Source: CAD feature listing. Evaluate the final solid. Frame: model axes, mm. A direction names the side the tool comes from. Give positions to 0.01 mm unless a question says otherwise; leave off trailing zeros. Write each loop counter-clockwise with the first axis right and the second up, starting at its lowest first coordinate (ties: lowest second). Pieces come first, ordered by that corner, then holes. Notation, with made-up numbers: (12.25, 60) -> (42.25, 60) arc R37 ccw to (42.25, 97) -> close; hole circle Ø1 at (49.25, 62). An arc over 180 degrees is marked (long way). Write item = value, one per line.
from build123d import *

# Parameters (mm, degrees)
SKETCH_2_W           = 80
SKETCH_2_H           = 34
SKETCH_2_R           = 4.05
EXTRUDE_1_DEPTH      = 8
SKETCH_3_R           = 2.55
CUT_EXTRUDE_1_DEPTH  = 88.292611371
CUT_EXTRUDE_2_DEPTH  = 88.292611371
SKETCH_5_R           = 1.55
CUT_EXTRUDE_3_DEPTH  = 88.292611371
CUT_EXTRUDE_15_DEPTH = 4.5
SKETCH_11_R          = 1.55
CUT_EXTRUDE_7_DEPTH  = 88.292611371
CUT_EXTRUDE_11_DEPTH = 2
SKETCH_21_R          = 2.9
CUT_EXTRUDE_13_DEPTH = 88.292611371
CUT_EXTRUDE_14_DEPTH = 6


with BuildPart() as part:
    # 草图2 → 凸台-拉伸1 (new body)
    with BuildSketch(Plane.XY):
        with Locations((40, 17)):
            Rectangle(SKETCH_2_W, SKETCH_2_H)
        with Locations((7, 8)):
            Circle(SKETCH_2_R, mode=Mode.SUBTRACT)
        with Locations((40, 10)):
            Circle(SKETCH_2_R, mode=Mode.SUBTRACT)
        with Locations((73, 8)):
            Circle(SKETCH_2_R, mode=Mode.SUBTRACT)
    extrude(amount=EXTRUDE_1_DEPTH)

    # 草图3 → 切除-拉伸1 (cut, through all)
    with BuildSketch(Plane.XY.offset(8)):
        with Locations((23, 8)):
            Circle(SKETCH_3_R)
        with Locations((57, 8)):
            Circle(SKETCH_3_R)
    extrude(amount=-CUT_EXTRUDE_1_DEPTH, mode=Mode.SUBTRACT)

    # 草图4 → 切除-拉伸2 (cut, through all)
    with BuildSketch(Plane(origin=(80, 0, 0), x_dir=(0, 0, -1), z_dir=(1, 0, 0))):
        Polygon((-1.5, 32.2), (-2.5, 32.2), (-2.5, 34), (0, 34), (0, 28.8), (-1.5, 28.8), align=None)
    extrude(amount=-CUT_EXTRUDE_2_DEPTH, mode=Mode.SUBTRACT)

    # 草图5 → 切除-拉伸3 (cut, through all)
    with BuildSketch(Plane.XY.offset(8)):
        with Locations((48, 10)):
            Circle(SKETCH_5_R)
        with Locations((32, 10)):
            Circle(SKETCH_5_R)
    extrude(amount=-CUT_EXTRUDE_3_DEPTH, mode=Mode.SUBTRACT)

    # 草图8 → 切除-拉伸15 (cut)
    with BuildSketch(Plane(origin=(0, 0, 0), x_dir=(-1, 0, 0), z_dir=(0, 0, -1))):
        Polygon((-48, 6.709103466), (-45.15, 8.354551733), (-45.15, 11.645448267), (-48, 13.290896534), (-50.85, 11.645448267), (-50.85, 8.354551733), align=None)
        Polygon((-34.85, 11.645448267), (-34.85, 8.354551733), (-32, 6.709103466), (-29.15, 8.354551733), (-29.15, 11.645448267), (-32, 13.290896534), align=None)
    extrude(amount=-CUT_EXTRUDE_15_DEPTH, mode=Mode.SUBTRACT)

    # 草图11 → 切除-拉伸7 (cut, through all)
    with BuildSketch(Plane(origin=(0, 0, 0), x_dir=(-1, 0, 0), z_dir=(0, 0, -1))):
        with Locations((-60, 25)):
            Circle(SKETCH_11_R)
        with Locations((-20, 25)):
            Circle(SKETCH_11_R)
    extrude(amount=-CUT_EXTRUDE_7_DEPTH, mode=Mode.SUBTRACT)

    # 草图19 → 切除-拉伸11 (cut)
    with BuildSketch(Plane(origin=(0, 0, 2.5), x_dir=(-1, 0, 0), z_dir=(0, 0, -1))):
        with BuildLine():
            Line((-25, 34), (-55.247938178, 34))
            Line((-55.247938178, 34), (-55.247938178, 33.2))
            ThreePointArc((-55.247938178, 33.2), (-54.747938178, 32.7), (-54.247938178, 33.2))
            Line((-54.247938178, 33.2), (-26, 33.2))
            ThreePointArc((-26, 33.2), (-25.5, 32.7), (-25, 33.2))
            Line((-25, 33.2), (-25, 34))
        make_face()
    extrude(amount=-CUT_EXTRUDE_11_DEPTH, mode=Mode.SUBTRACT)

    # 草图21 → 切除-拉伸13 (cut, through all)
    with BuildSketch(Plane(origin=(0, 0, 0), x_dir=(-1, 0, 0), z_dir=(0, 0, -1))):
        with Locations((-66.5, 11.5)):
            Circle(SKETCH_21_R)
        with Locations(Location((-13.5, 11.5, 0), (0, 0, 180))):
            Circle(SKETCH_21_R)
    extrude(amount=-CUT_EXTRUDE_13_DEPTH, mode=Mode.SUBTRACT)

    # 草图22 → 切除-拉伸14 (cut)
    with BuildSketch(Plane(origin=(0, 0, 0), x_dir=(-1, 0, 0), z_dir=(0, 0, -1))):
        Polygon((-52.9, 5.632863896), (-52.9, 10.367136104), (-57, 12.734272207), (-61.1, 10.367136104), (-61.1, 5.632863896), (-57, 3.265727793), align=None)
        Polygon((-23, 3.265727793), (-18.9, 5.632863896), (-18.9, 10.367136104), (-23, 12.734272207), (-27.1, 10.367136104), (-27.1, 5.632863896), align=None)
    extrude(amount=-CUT_EXTRUDE_14_DEPTH, mode=Mode.SUBTRACT)


solid = part.part
1) Material intervals for L1, parallel to Y at x = 60, z = 2; L2, parallel to Y at x = 32, z = 5.45; L3, parallel to X at y = 6.5, z = 7, sorted ascending.
Computed:
L1 = 0 to 5, 11 to 23.45, 26.55 to 32.2
L2 = 0 to 8.45, 11.55 to 34
L3 = 0 to 3.24, 10.76 to 20.94, 25.06 to 37.96, 42.04 to 54.94, 59.06 to 69.24, 76.76 to 80
2) Draft query along X for faces 1 (the flat face through (39, 34, 5)), 2 (the flat face through (0, 17, 4)), 3 (the flat face through (33.405, 12.48, 2.218)). Return one class per face: pulls with the +X half, pulls with the -X half, needs draft (parallel to the pull), parting line crosses it, or undercut.
Computed:
face_1 = needs draft
face_2 = pulls with the -X half
face_3 = undercut
3) Cut plane C-C (x = 73). Return the cut outline in (y, z).
Computed:
outline = (0, 0) -> (3.95, 0) -> (3.95, 8) -> (0, 8) -> close; (12.05, 0) -> (28.8, 0) -> (28.8, 1.5) -> (32.2, 1.5) -> (32.2, 2.5) -> (34, 2.5) -> (34, 8) -> (12.05, 8) -> close
4) Access query for faces 4 (the cylindrical face through (54.452, 8.112, 7.014)), 5 (the flat face through (30.595, 7.52, 2.218)). Directions: +Z, -Z, +X, -X, +Y, -Y. A direction counts if a zero-diameter tool reaches every point of the face in a straight line with its end or side. Return the directions, or none.
Computed:
face_4 = +Z, -Z
face_5 = -Z
5) Cut plane A-A (x = 13.5). Return the cut outline in (y, z).
Computed:
outline = (0, 0) -> (8.6, 0) -> (8.6, 8) -> (0, 8) -> close; (14.4, 0) -> (28.8, 0) -> (28.8, 1.5) -> (32.2, 1.5) -> (32.2, 2.5) -> (34, 2.5) -> (34, 8) -> (14.4, 8) -> close
6) Cut plane D-D (y = 31.5). Return the cut outline in (x, z), then the cut area to 3 significant figures.
Computed:
outline = (0, 1.5) -> (80, 1.5) -> (80, 8) -> (0, 8) -> close
area = 520 mm²
7) Contact query for flat-ended pins moving along their axis: pin 1 (2.5 mm diameter, centred on x = 23, y = 10, fed in from -Z); pin 2 (1.7 mm diameter, centred on x = 48.5, y = 8.5, fed in from -Z); pin 3 (1 mm diameter, centred on x = 39.5, y = 33.5, fed in from -Z). Output: stop coordinate, or through.
Computed:
pin_1 = 6
pin_2 = 4.5
pin_3 = 2.5
8) Cut plane B-B (z = 6.75). State how many separate pieces and enclosed holes the cut face has, then the cut area to 3 significant figures.
Computed:
separate_pieces = 1
enclosed_holes = 11
area = 2,440 mm²
